Could you check a few things on this model? Use its own coordinates, in mm. Face numbers are marked on the shaded views. A direction names the side the tool comes from. Round coordinates to 2 decimals unless told otherwise and drop trailing zeros. Loops run counter-clockwise (first coordinate to the right, second up) from the corner with the lowest first, then second, coordinate; pieces in that order, holes last. Notation, with made-up numbers: (-10, 22.5) - (8, 22.5) arc R21 cw to (8, 50.5) - close; hole circle Ø11 at (-20.75, -29). An arc over 180 degrees is marked (long way). Use one line per item in the form item = value.
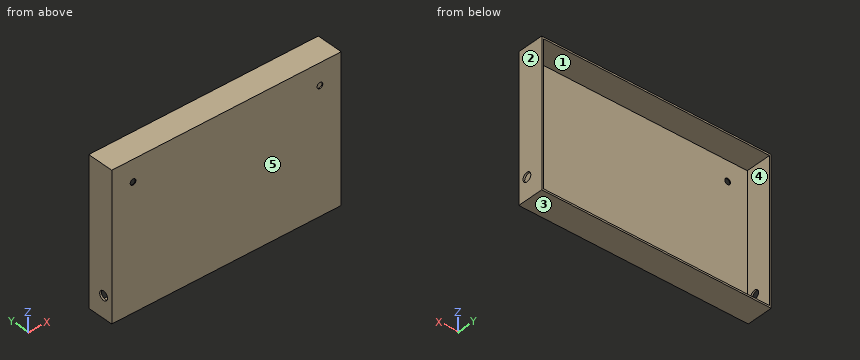
```python
from build123d import *

# Parameters (mm, degrees)
SKETCH2_W           = 269
SKETCH2_H           = 169
SKETCH2_W_2         = 265
SKETCH2_H_2         = 165
WALLS_DEPTH         = 30
SKETCH2_2_W         = 269
SKETCH2_2_H         = 169
SKETCH2_2_W_2       = 265
SKETCH2_2_H_2       = 165
BASE_DEPTH          = 1
SKETCH4_R           = 5.25
MOTOR_WHEEL_DEPTH   = 10
MOTOR_WHEEL2_START  = -10
SKETCH3_R           = 5.25
MOTOR_WHEEL2_DEPTH  = 10
SKETCH6_R           = 3.35
CASTER_WHEELS_DEPTH = 10


with BuildPart() as part:
    # Sketch2 → Walls (new body)
    with BuildSketch(Plane(origin=(0, 0, 0), x_dir=(1, 0, 0), z_dir=(0, 1, 0))):
        with Locations((64.006127086, -35.704235294)):
            Rectangle(SKETCH2_W, SKETCH2_H)
        with Locations((64.006127086, -35.704235294)):
            Rectangle(SKETCH2_W_2, SKETCH2_H_2, mode=Mode.SUBTRACT)
    extrude(amount=WALLS_DEPTH)

    # Sketch2_2 → Base (add)
    # profile 1 of 2: a face of its own
    with BuildSketch(Plane(origin=(0, 0, 0), x_dir=(1, 0, 0), z_dir=(0, 1, 0))):
        with Locations((64.006127086, -35.704235294)):
            Rectangle(SKETCH2_2_W, SKETCH2_2_H)
        with Locations((64.006127086, -35.704235294)):
            Rectangle(SKETCH2_2_W_2, SKETCH2_2_H_2, mode=Mode.SUBTRACT)
    # profile 2 of 2: a face of its own
    with BuildSketch(Plane(origin=(0, 0, 0), x_dir=(1, 0, 0), z_dir=(0, 1, 0))):
        with Locations((64.006127086, -35.704235294)):
            Rectangle(SKETCH2_2_W_2, SKETCH2_2_H_2)
    extrude(amount=-BASE_DEPTH)

    # Sketch4 → Motor-Wheel (cut)
    with BuildSketch(Plane(origin=(198.506127086, 0, 0), x_dir=(0, 0, -1), z_dir=(1, 0, 0))):
        with Locations((23.795764706, 10)):
            Circle(SKETCH4_R)
    extrude(amount=-MOTOR_WHEEL_DEPTH, mode=Mode.SUBTRACT)

    # Sketch3 → Motor-Wheel2 (cut)
    with BuildSketch(Plane.ZY.offset(70.493872914).offset(MOTOR_WHEEL2_START)):
        with Locations(Location((-23.795764706, 10, 0), (0, 0, 180))):
            Circle(SKETCH3_R)
    extrude(amount=MOTOR_WHEEL2_DEPTH, mode=Mode.SUBTRACT)

    # Sketch6 → Caster Wheels (cut)
    with BuildSketch(Plane(origin=(0, 0, 0), x_dir=(1, 0, 0), z_dir=(0, 1, 0))):
        with Locations(Location((-45.493872914, -95.204235294, 0), (0, 0, 270))):
            Circle(SKETCH6_R)
        with Locations(Location((173.506127086, -95.204235294, 0), (0, 0, 270))):
            Circle(SKETCH6_R)
    extrude(amount=-CASTER_WHEELS_DEPTH, mode=Mode.SUBTRACT)


solid = part.part
```
1. If we section it at C-C, the plane y = 23: Write out the boundary of the cut face in (x, z), plus the area to 3 significant figures.
Solution:
outline = (-70.49, -48.8) - (198.51, -48.8) - (198.51, 120.2) - (-70.49, 120.2) - close; hole (-68.49, -46.8) - (196.51, -46.8) - (196.51, 118.2) - (-68.49, 118.2) - close
area = 1,740 mm^2
2. If we section it at A-A, the plane y = 10: Write out the boundary of the cut face in (x, z).
Solution:
outline = (-70.49, -48.8) - (198.51, -48.8) - (198.51, -29.05) - (196.51, -29.05) - (196.51, -46.8) - (-68.49, -46.8) - (-68.49, -29.05) - (-70.49, -29.05) - close; (-70.49, -18.55) - (-68.49, -18.55) - (-68.49, 118.2) - (196.51, 118.2) - (196.51, -18.55) - (198.51, -18.55) - (198.51, 120.2) - (-70.49, 120.2) - close
3. For P1, Ø3, axis at x = 82.5, z = 95, coming from the +Y side; P2, Ø10.5, axis at x = -45.49, z = 95.2, coming from the -Y side, each with a flat end and sliding along its axis, tell me the tip position at first contact or that it passes through.
Solution:
P1 = 0
P2 = -1
4. If we section it at B-B, the plane z = 15: Write out the boundary of the cut face in (x, y), plus the area to 3 significant figures.
Solution:
outline = (-70.49, -1) - (198.51, -1) - (198.51, 30) - (196.51, 30) - (196.51, 0) - (-68.49, 0) - (-68.49, 30) - (-70.49, 30) - close
area = 389 mm^2
5. If we section it at D-D, the plane x = 54.5: Write out the boundary of the cut face in (y, z).
Solution:
outline = (-1, -48.8) - (30, -48.8) - (30, -46.8) - (0, -46.8) - (0, 118.2) - (30, 118.2) - (30, 120.2) - (-1, 120.2) - close
6. We'd pull the mould along Z, two halves only. Please class the marked faces 3, 4 and 5: +Z half, -Z half, draft (parallel to the pull), parting line (faces both ways), or undercut.
Solution:
face_3 = -Z half
face_4 = undercut
face_5 = draft
7. Please list where these lines run through material, in increasing order: line 1 along Z through (x, y) = (183.5, 16); line 2 along X through (y, z) = (28.5, -7); line 3 along Z through (x, y) = (-69, 10).
Solution:
line_1 = -48.8 to -46.8, 118.2 to 120.2
line_2 = -70.49 to -68.49, 196.51 to 198.51
line_3 = -48.8 to -29.05, -18.55 to 120.2
8. On a 3-axis mill with a long thin cutter (end or side, diameter ignored), from which of +Z, -Z, +X, -X, +Y, -Y can I reach the whole of each face in a straight line? I mean the marked faces 1 and 2. Say none if no direction works.
Solution:
face_1 = +Y
face_2 = +Z, -Z, +X, +Y, -Y
